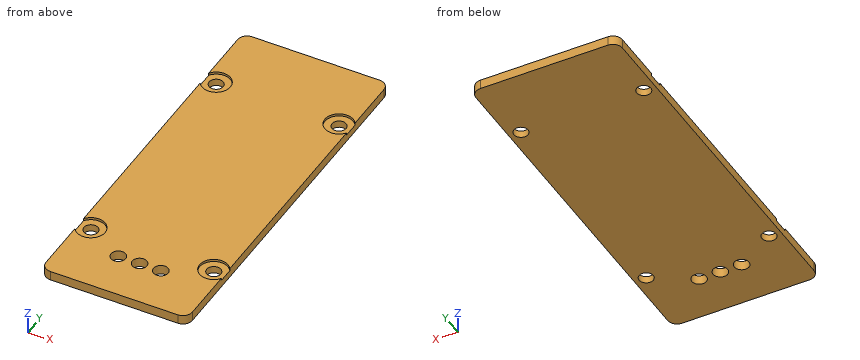
from build123d import *

# Parameters (mm, degrees)
PAD_DEPTH       = 2
SKETCH001_R     = 1.5
POCKET_DEPTH    = 2.001
SKETCH002_R     = 3
POCKET001_DEPTH = 0.5
SKETCH003_R     = 1.55
POCKET002_DEPTH = 2.001
FILLET_R        = 2


with BuildPart() as part:
    # Sketch → Pad (new body)
    with BuildSketch(Plane.XY):
        Polygon((0, 0), (15.5, 0), (15.5, 39.5), (15.5, 79), (0, 79), (-15.5, 79), (-15.5, 39.5), (-15.5, 0), align=None)
    extrude(amount=PAD_DEPTH)

    # Sketch001 (on DatumPlane) → Pocket (cut, through all)
    with BuildSketch(Plane(origin=(0, 0, 2), x_dir=(-1, 0, 0), z_dir=(0, 0, 1))):
        with Locations((-13, -15)):
            Circle(SKETCH001_R)
        with Locations((13, -15)):
            Circle(SKETCH001_R)
        with Locations((-13, -64)):
            Circle(SKETCH001_R)
        with Locations((13, -64)):
            Circle(SKETCH001_R)
    extrude(amount=-POCKET_DEPTH, mode=Mode.SUBTRACT)

    # Sketch002 (on DatumPlane) → Pocket001 (cut)
    with BuildSketch(Plane(origin=(0, 0, 2), x_dir=(-1, 0, 0), z_dir=(0, 0, 1))):
        with Locations((-13, -15)):
            Circle(SKETCH002_R)
        with Locations((13, -15)):
            Circle(SKETCH002_R)
        with Locations((-13, -64)):
            Circle(SKETCH002_R)
        with Locations((13, -64)):
            Circle(SKETCH002_R)
    extrude(amount=-POCKET001_DEPTH, mode=Mode.SUBTRACT)

    # Sketch003 (on DatumPlane) → Pocket002 (cut, through all)
    with BuildSketch(Plane(origin=(0, 0, 2), x_dir=(-1, 0, 0), z_dir=(0, 0, 1))):
        with Locations((0, -10)):
            Circle(SKETCH003_R)
        with Locations((-4.5, -10)):
            Circle(SKETCH003_R)
        with Locations((4.5, -10)):
            Circle(SKETCH003_R)
    extrude(amount=-POCKET002_DEPTH, mode=Mode.SUBTRACT)

    # Fillet
    fillet_edges = [part.edges().sort_by_distance(p)[0] for p in [
        (15.5, 79, 1),
        (-15.5, 79, 1),
        (-15.5, 0, 1),
        (15.5, 0, 1),
    ]]
    fillet(fillet_edges, radius=FILLET_R)


solid = part.part
Model file for the job. Use its own axes, mm. Round coordinates to 2 decimals unless told otherwise and drop trailing zeros. Order: outer loops, then holes, each group sorted by start corner. A loop starts at its lowest first (then second) coordinate and runs counter-clockwise, first axis right, second up. Notation, with made-up numbers: M -6,-27 L 45,-27 A23 cw 45,-10 Z; hole C -34,63.5 d2. An arc over 180 degrees is marked long. Write each question's results on one line, items separated by ' | '. Start each with the question number.
(1) Saw through at B-B, the plane y = 64. Give the cut face in (x, z), then the cut area to 3 significant figures.
(2) Saw through at C-C, the plane z = 0.7. Give the cut face in (x, y).
(3) Probe probe 1 along Y at (x, z) = (13, 1); probe 2 along Y at (x, z) = (-13, 1.8); probe 3 along X at (y, z) = (10, 1.3). List the from-to ranges inside material, lowest first. Write a range as from..to.
(4) Saw through at A-A, the plane x = 4.5. Give the cut face in (y, z), then the cut area to 3 significant figures.
(5) Saw through at D-D, the plane y = 10. Give the cut face in (x, z), then the cut area to 3 significant figures.
(6) Drop flat-ended pins along their axis: pin 1 (12 mm diameter, centred on x = -8.5, y = 41, fed in from -Z); pin 2 (3 mm diameter, centred on x = -14, y = 63, fed in from +Z). Give the stop position or say it passes through.
Established:
1) outline: M -15.5,0 L -14.5,0 L -14.5,1.5 L -15.5,1.5 Z; M -11.5,0 L 11.5,0 L 11.5,1.5 L 10,1.5 L 10,2 L -10,2 L -10,1.5 L -11.5,1.5 Z; M 14.5,0 L 15.5,0 L 15.5,1.5 L 14.5,1.5 Z | area: 47.5 mm^2
2) outline: M -15.5,2 A2 ccw -13.5,0 L 13.5,0 A2 ccw 15.5,2 L 15.5,77 A2 ccw 13.5,79 L -13.5,79 A2 ccw -15.5,77 Z; hole C -13,15 d3; hole C -13,64 d3; hole C -4.5,10 d3.1; hole C 0,10 d3.1; hole C 4.5,10 d3.1; hole C 13,15 d3; hole C 13,64 d3
3) probe 1: y = 0..13.5, 16.5..62.5, 65.5..79 | probe 2: y = 0..12, 18..61, 67..79 | probe 3: x = -15.5..-6.05, -2.95..-1.55, 1.55..2.95, 6.05..15.5
4) outline: M 0,0 L 8.45,0 L 8.45,2 L 0,2 Z; M 11.55,0 L 79,0 L 79,2 L 11.55,2 Z | area: 152 mm^2
5) outline: M -15.5,0 L -6.05,0 L -6.05,2 L -15.5,2 Z; M -2.95,0 L -1.55,0 L -1.55,2 L -2.95,2 Z; M 1.55,0 L 2.95,0 L 2.95,2 L 1.55,2 Z; M 6.05,0 L 15.5,0 L 15.5,2 L 6.05,2 Z | area: 43.4 mm^2
6) pin 1: stops at z = 0 | pin 2: stops at z = 1.5
